The model under review builds one solid part; all positions refer to its coordinate system, in mm. Face numbers are marked on the shaded views. A direction names the side the tool comes from. Round coordinates to 2 decimals unless told otherwise and drop trailing zeros. Write each loop counter-clockwise with the first axis right and the second up, starting at its lowest first coordinate (ties: lowest second). Pieces come first, ordered by that corner, then holes. Notation, with made-up numbers: M 55,55 L 109,55 A27 cw 109,74 Z; hole C 13.5,19.5 d6. An arc over 180 degrees is marked long. Write item = value, one per line. Start each with the question number.
Item 1: Take a section at A-A, the plane y = 12. Give the boundary of the cut face in (x, z).
Item 2: For pin 1 Ø2 at (x, z) = (-13, 3.5) entering from -Y; pin 2 Ø5 at (y, z) = (-2.5, 4.5) entering from +X; pin 3 Ø2 at (y, z) = (0, 8) entering from +X, all flat-tipped, find the tip position at first contact; note any pin that passes through.
Item 3: The part is to be moulded in two halves that separate along X. For the marked faces 1, 2 and 3, say which applies: +X half, -X half, draft (parallel to the pull), parting line (faces both ways), or undercut.
Item 4: Take a section at C-C, the plane x = 61. Give the boundary of the cut face in (y, z), plus the area to 3 significant figures.
Item 5: To check wall thickness, follow line 1 along Y through (x, z) = (2.5, 1); line 2 along X through (y, z) = (-31.5, 6.25); line 3 along X through (y, z) = (8, 5.25). State the ranges of each line that lie inside material, in increasing order.
Item 6: Take a section at B-B, the plane x = -28. Give the boundary of the cut face in (y, z), plus the area to 3 significant figures.
Item 7: Tool access review of the marked faces 4 and 5: name each direction out of +Z, -Z, +X, -X, +Y, -Y from which nothing blocks a thin tool from reaching the whole face with its end or side.
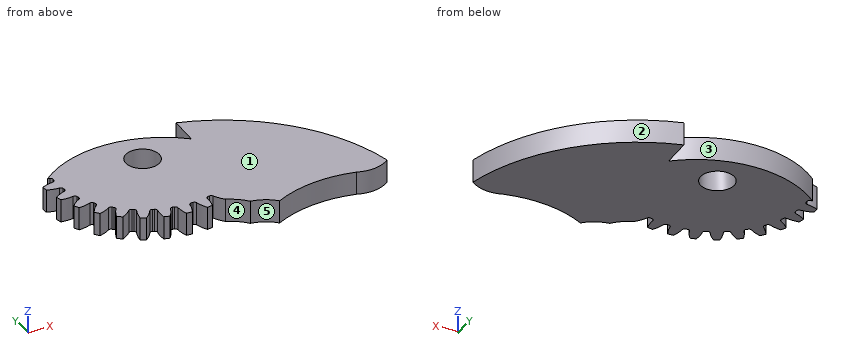
from build123d import *

# Parameters (mm, degrees)
SKETCH3_R               = 40.64
GEARBODY_DEPTH          = 25.4
TOOTHCUT_DEPTH          = 63.836129734
CIRPATTERN1_COUNT       = 30
BOREDIA_R               = 9.525
BORE_DEPTH              = 12700
CUT_EXTRUDE1_DEPTH      = 63.817881856
BOSS_EXTRUDE1_DEPTH     = 25.4
CUT_EXTRUDE2_DEPTH      = 97.248090867
CUT_EXTRUDE2_DEPTH_BACK = 97.248090867
CUT_EXTRUDE3_DEPTH      = 94.297837255
CUT_EXTRUDE3_DEPTH_BACK = 94.297837255
SKETCH8_R               = 10.901188975
SKETCH8_R_2             = 6.746875
BOSS_EXTRUDE2_DEPTH     = 9.271
CUT_EXTRUDE4_DEPTH      = 94.297837255
CUT_EXTRUDE4_DEPTH_BACK = 94.297837255


with BuildPart() as part:
    # Sketch3 → gearBody (new body)
    with BuildSketch(Plane.XY):
        Circle(SKETCH3_R)
    extrude(amount=GEARBODY_DEPTH)

    # Sketch2 → toothCut (cut, through all)
    with BuildSketch(Plane.XY):
        with BuildLine():
            ThreePointArc((34.901466352, -2.640387833), (34.929801576, -2.234493965), (34.953416534, -1.828298136))
            ThreePointArc((34.953416534, -1.828298136), (35.218972856, -1.205360668), (35.823821616, -0.900845929))
            ThreePointArc((35.823821616, -0.900845929), (41.902420255, 1.180053047), (46.567899911, 5.597382731))
            ThreePointArc((46.567899911, 5.597382731), (46.807414621, -2.994316622), (45.4750933, -11.485464069))
            ThreePointArc((45.4750933, -11.485464069), (41.410501506, -6.509663078), (35.646600115, -3.671187658))
            ThreePointArc((35.646600115, -3.671187658), (35.08548304, -3.292084932), (34.901466352, -2.640387833))
        make_face()
    toothcut = extrude(amount=TOOTHCUT_DEPTH, mode=Mode.SUBTRACT)

    # CirPattern1: toothCut ×30 about axis
    cirpattern1_axis = Axis((0, 0, 0), (0, 0, 1))
    for i in range(1, CIRPATTERN1_COUNT):
        add(toothcut.rotate(cirpattern1_axis, i * 360 / CIRPATTERN1_COUNT), mode=Mode.SUBTRACT)

    # boreDia → bore (cut, symmetric)
    with BuildSketch(Plane.XY):
        Circle(BOREDIA_R)
    extrude(amount=BORE_DEPTH, both=True, mode=Mode.SUBTRACT)

    # Sketch4 → Cut-Extrude1 (cut, through all)
    with BuildSketch(Plane.XY.offset(25.4)):
        with BuildLine():
            ThreePointArc((-43.554352266, 3.655257975), (1.299887875, 18.694416006), (46.382242057, 4.353548725))
            ThreePointArc((46.382242057, 4.353548725), (1.078287813, 47.235471327), (-43.554352266, 3.655257975))
        make_face()
    extrude(amount=-CUT_EXTRUDE1_DEPTH, mode=Mode.SUBTRACT)

    # Sketch5 → Boss-Extrude1 (add)
    with BuildSketch(Plane.XY.offset(25.4)):
        with BuildLine():
            Line((-40.520407877, 5.797825642), (17.717099168, 12.48871132))
            Line((17.717099168, 12.48871132), (8.960832095, -26.928019276))
            Line((8.960832095, -26.928019276), (13.028048789, -38.495188592))
            ThreePointArc((13.028048789, -38.495188592), (20.295398902, -43.922390287), (24.158608262, -52.128760334))
            ThreePointArc((24.158608262, -52.128760334), (42.8096102, -43.78426266), (63.240034891, -44.081351255))
            ThreePointArc((63.240034891, -44.081351255), (70.340218446, -44.816365594), (76.818795497, -41.819551953))
            ThreePointArc((76.818795497, -41.819551953), (30.86783196, 13.330528242), (-40.520407877, 5.797825642))
        make_face()
    extrude(amount=-BOSS_EXTRUDE1_DEPTH)

    # Sketch6 → Cut-Extrude2 (cut, two sides: drawn at the far end of the back side and taken through both)
    with BuildSketch(Plane(origin=(0, 0, 0), x_dir=(1, 0, 0), z_dir=(0, 1, 0)).offset(-CUT_EXTRUDE2_DEPTH_BACK)):
        Polygon((-46.138376309, -9.271), (97.816171298, -9.271), (71.932802696, -41.15378122), (-48.678279579, -38.064709676), align=None)
    extrude(amount=CUT_EXTRUDE2_DEPTH + CUT_EXTRUDE2_DEPTH_BACK, mode=Mode.SUBTRACT)

    # Sketch7 → Cut-Extrude3 (cut, two sides: drawn at the far end of the back side and taken through both)
    with BuildSketch(Plane.XY.offset(9.271).offset(-CUT_EXTRUDE3_DEPTH_BACK)):
        with BuildLine():
            Line((21.841106952, 3.893976142), (22.251299285, 16.241253613))
            Line((22.251299285, 16.241253613), (23.901139449, 23.204831581))
            Line((23.901139449, 23.204831581), (-36.876630256, 21.261551183))
            Line((-36.876630256, 21.261551183), (-43.577597148, 3.302959913))
            Line((-43.577597148, 3.302959913), (-36.448484964, 3.893976142))
            ThreePointArc((-36.448484964, 3.893976142), (-7.303689006, 14.730432769), (21.841106952, 3.893976142))
        make_face()
    extrude(amount=CUT_EXTRUDE3_DEPTH + CUT_EXTRUDE3_DEPTH_BACK, mode=Mode.SUBTRACT)

    # Sketch8 → Boss-Extrude2 (add)
    with BuildSketch(Plane.XY.offset(9.271)):
        Circle(SKETCH8_R)
        Circle(SKETCH8_R_2, mode=Mode.SUBTRACT)
    extrude(amount=-BOSS_EXTRUDE2_DEPTH)

    # Sketch9 → Cut-Extrude4 (cut, two sides: drawn at the far end of the back side and taken through both)
    with BuildSketch(Plane.XY.offset(9.271).offset(-CUT_EXTRUDE4_DEPTH_BACK)):
        with BuildLine():
            Line((20.295398902, -43.922390287), (23.1683449, -52.694459817))
            Line((23.1683449, -52.694459817), (26.579367988, -52.803988081))
            Line((26.579367988, -52.803988081), (29.661056762, -48.607867727))
            ThreePointArc((29.661056762, -48.607867727), (25.399491401, -45.423078115), (20.295398902, -43.922390287))
        make_face()
    extrude(amount=CUT_EXTRUDE4_DEPTH + CUT_EXTRUDE4_DEPTH_BACK, mode=Mode.SUBTRACT)


solid = part.part
Response values:
q1.outline = M -22.67,0 L 8.06,0 L 8.06,9.27 L -22.67,9.27 Z; M 22.11,0 L 33.95,0 L 33.95,9.27 L 22.11,9.27 Z
q2.pin_1 = -38.83
q2.pin_2 = 57.65
q2.pin_3 = 53.59
q3.face_1 = draft
q3.face_2 = +X half
q3.face_3 = undercut
q4.outline = M -43.61,0 L -8.8,0 L -8.8,9.27 L -43.61,9.27 Z
q4.area = 323 mm2
q5.line_1 = -35.17 to -6.27, 6.27 to 13.64
q5.line_2 = -25.68 to -24.1, -19.06 to 73.91
q5.line_3 = -30.87 to 16.26, 21.98 to 41.52
q6.outline = M -24.88,0 L 9.64,0 L 9.64,9.27 L -24.88,9.27 Z
q6.area = 320 mm2
q7.face_4 = +Z, -Z, -Y
q7.face_5 = +Z, -Z, -X, -Y
